from build123d import *

# Parameters (mm, degrees)
ESQUISSE1_R             = 56
ESQUISSE1_R_2           = 38
BOSS_EXTRU_1_DEPTH      = 11
ESQUISSE2_R             = 4.25
ENL_V_MAT_EXTRU_2_DEPTH = 11
ESQUISSE2_5_R           = 4.25
ENL_V_MAT_EXTRU_3_DEPTH = 12
CONG_1_R                = 1
CONG_2_R                = 1


with BuildPart() as part:
    # Esquisse1 → Boss.-Extru.1 (new body)
    with BuildSketch(Plane.XY):
        Circle(ESQUISSE1_R)
        Circle(ESQUISSE1_R_2, mode=Mode.SUBTRACT)
    extrude(amount=BOSS_EXTRU_1_DEPTH)

    # Esquisse2 → Enl_v. mat.-Extru.2 (cut)
    with BuildSketch(Plane.XY.offset(11)):
        with Locations((0, 47)):
            Circle(ESQUISSE2_R)
    extrude(amount=-ENL_V_MAT_EXTRU_2_DEPTH, mode=Mode.SUBTRACT)

    # Esquisse2_5 → Enl_v. mat.-Extru.3 (cut, through all)
    with BuildSketch(Plane.XY.offset(11)):
        with Locations((0, 47)):
            Circle(ESQUISSE2_5_R)
        with Locations((0, -47)):
            Circle(ESQUISSE2_5_R)
        with Locations((40.703193978, -23.5)):
            Circle(ESQUISSE2_5_R)
        with Locations((40.703193978, 23.5)):
            Circle(ESQUISSE2_5_R)
        with Locations((-40.703193978, 23.5)):
            Circle(ESQUISSE2_5_R)
        with Locations((-40.703193978, -23.5)):
            Circle(ESQUISSE2_5_R)
    extrude(amount=-ENL_V_MAT_EXTRU_3_DEPTH, mode=Mode.SUBTRACT)

    # Cong_1
    cong_1_edges = [part.edges().sort_by_distance(p)[0] for p in [
        (-56, 0, 11),
    ]]
    fillet(cong_1_edges, radius=CONG_1_R)

    # Cong_2
    cong_2_edges = [part.edges().sort_by_distance(p)[0] for p in [
        (-56, 0, 0),
    ]]
    fillet(cong_2_edges, radius=CONG_2_R)


solid = part.part
Verification items for the finished model (mm, model axes). Coordinates: 2 decimals unless noted, no trailing zeros. Write each loop counter-clockwise with the first axis right and the second up, starting at its lowest first coordinate (ties: lowest second). Pieces come first, ordered by that corner, then holes. Notation, with made-up numbers: M 43,20.25 L 65,20.25 A28 cw 65,54.25 Z; hole C -32.5,8.25 d6. An arc over 180 degrees is marked long. Use a Markdown table: item, result.
Q1. Sectioned sample at D-D, the plane x = -40.5. Count the separate pieces of the cut face and the enclosed holes in it, plus the area to 3 significant figures.
Reply:
| item | result |
|---|---|
| separate pieces | 3 |
| enclosed holes | 0 |
| area | 663 mm² |
Q2. Sectioned sample at B-B, the plane x = 0. Record the boundary of the cut face in (y, z), plus the area to 3 significant figures.
Reply:
| item | result |
|---|---|
| outline | M -56,1 A1 ccw -55,0 L -51.25,0 L -51.25,11 L -55,11 A1 ccw -56,10 Z; M -42.75,0 L -38,0 L -38,11 L -42.75,11 Z; M 38,0 L 42.75,0 L 42.75,11 L 38,11 Z; M 51.25,0 L 55,0 A1 ccw 56,1 L 56,10 A1 ccw 55,11 L 51.25,11 Z |
| area | 208 mm² |
Q3. Sectioned sample at A-A, the plane y = 0. Record the boundary of the cut face in (x, z), plus the area to 3 significant figures.
Reply:
| item | result |
|---|---|
| outline | M -56,1 A1 ccw -55,0 L -38,0 L -38,11 L -55,11 A1 ccw -56,10 Z; M 38,0 L 55,0 A1 ccw 56,1 L 56,10 A1 ccw 55,11 L 38,11 Z |
| area | 395 mm² |
Q4. Thickness scan on line 1 (Y direction, x = 0, z = 5.5); line 2 (Y direction, x = -40, z = 2.5); line 3 (Y direction, x = -31.5, z = 7.75). Record the ranges inside material, lowest first.
Reply:
| item | result |
|---|---|
| line 1 | y = -56 to -51.25, -42.75 to -38, 38 to 42.75, 51.25 to 56 |
| line 2 | y = -39.19 to -27.69, -19.31 to 19.31, 27.69 to 39.19 |
| line 3 | y = -46.3 to -21.25, 21.25 to 46.3 |
Q5. Draft check along Y on faces 1 (the face through (51.73, -21.45, 5.44)), 2 (the face through (-44.95, 23.69, 5.58)), 3 (the face through (36, 13, 0)). Enter one of: +Y half, -Y half, draft (parallel to the pull), parting line (faces both ways), or undercut.
Reply:
| item | result |
|---|---|
| face 1 | parting line |
| face 2 | undercut |
| face 3 | draft |
Q6. Sectioned sample at C-C, the plane z = 2.75. Record the boundary of the cut face in (x, y), plus the area to 3 significant figures.
Reply:
| item | result |
|---|---|
| outline | C 0,0 d112; hole C -40.7,-23.5 d8.5; hole C -40.7,23.5 d8.5; hole C 0,0 d76; hole C 0,-47 d8.5; hole C 0,47 d8.5; hole C 40.7,-23.5 d8.5; hole C 40.7,23.5 d8.5 |
| area | 4,980 mm² |
Q7. Go/stop test with flat-tipped pins: P1, Ø2, axis at y = 19.5, z = 8.5, coming from the -X side; P2, Ø7, axis at x = 40.7, y = 23.5, coming from the +Z side; P3, Ø1, axis at x = -2, z = 4, coming from the +Y side; P4, Ø6, axis at x = 18.5, z = 9.5, coming from the -Y side. Record where each tip stops, or that it passes through.
Reply:
| item | result |
|---|---|
| P1 | stops at x = -52.86 |
| P2 | passes through |
| P3 | stops at y = 55.98 |
| P4 | stops at y = -53.81 |
